Source: CAD feature listing. Evaluate the final solid. Frame: model axes, mm. A direction names the side the tool comes from. Give positions to 0.01 mm unless a question says otherwise; leave off trailing zeros. Write each loop counter-clockwise with the first axis right and the second up, starting at its lowest first coordinate (ties: lowest second). Pieces come first, ordered by that corner, then holes. Notation, with made-up numbers: (57, -23) -> (65, -23) arc R23 cw to (65, -14) -> close; hole circle Ø1 at (83.5, 21). An arc over 180 degrees is marked (long way). Answer as a JSON object with one key per item and string values. Group by question number.
Item 1: First-contact query: pin 1 Ø4 at (x, z) = (714, 304.5) entering from +Y; pin 2 Ø1.5 at (x, y) = (726, 437) entering from -Z; pin 3 Ø8 at (x, z) = (572, 173) entering from +Y. Flat tips, straight axial feed; report the tip coordinate or a pass-through.
Item 2: Access query for faces 1 (the face through (688.11, 629.81, -443.7)), 2 (the face through (687, 638, -900)). Directions: +Z, -Z, +X, -X, +Y, -Y. A direction counts if a zero-diameter tool reaches every point of the face in a straight line with its end or side. Return the directions, or none.
Item 3: Ray query, probe 1 along Z at (x, y) = (528, 589.5); probe 2 along Z at (x, y) = (235, 513.5); probe 3 along X at (y, z) = (640.5, -573.5). Return the intervals inside material, ascending. Write a range as from..to.
Item 4: Section query A-A on z = -118. Return the cut outline in (x, y), plus the area to 3 significant figures.
Autodesk Inventor part; units mm, degrees
ref_plane "end1" through (-1039.2305, 0, 0) normal (1, 0, 0) x (0, 1, 0)
ref_plane "end2" through (1039.2305, 0, 0) normal (1, 0, 0) x (0, 1, 0)
ref_plane "XZ Plane" through (0, 0, 0) normal (0, 1, 0) x (-1, 0, 0)
sketch "Sketch1" plane through (0, 0, 0) normal (0, 0, 1) x (1, 0, 0)
  arc A0 (0, 900) -> (-1039.2305, 0) centre (0, -150) ccw
  arc A1 (1039.2305, 0) -> (0, 900) centre (0, -150) ccw
  arc A2 (0, 890) -> (-1029.1258, 0) centre (0, -150) ccw
  arc A3 (1029.1258, 0) -> (0, 890) centre (0, -150) ccw
  line L0 (1029.1258, 0) -> (1039.2305, 0)
  line L1 (-1039.2305, 0) -> (-1029.1258, 0)
  point P0 (0, 0)
  dimension "d0" = 0
  dimension "d1" = 0
  dimension "d2" = 0
  dimension "d3" = 150
  dimension "d6" = 900
  dimension "d8" = 1039.2305
  dimension "d10" = 0
  dimension "d11" = 10
  dimension "d12" = 0
revolve "Revolution2" add sketch "Sketch1" angle 90 about axis through (1029.1258, 0, 0) along (1, 0, 0)
ref_plane "end1" through (-1039.2305, 0, 0) normal (1, 0, 0) x (0, 1, 0)
sketch "Sketch3" plane through (-1039.2305, 0, 0) normal (1, 0, 0) x (0, 1, 0)
  line L0 (900, 0) -> (0, 0)
  line L1 (0, 900) -> (0, 0)
  line L2 (900, 0) -> (0, 0)
  line L3 (0, 0) -> (0, 900)
  line L4 (0, 900) -> (900, 900)
  line L5 (900, 900) -> (900, 0)
extrude "Extrusion1" cut sketch "Sketch3" along normal blind 1039.2305
ref_plane "end2" through (1039.2305, 0, 0) normal (1, 0, 0) x (0, 1, 0)
sketch "Sketch4" plane through (0, -150, 0) normal (0, 0, -1) x (-0.7559289, 0.6546537, 0)
  arc A0 (687.3864, 793.7254) -> (-687.3864, 793.7254) centre (0, 0) ccw
  arc A1 (680.8398, 786.1661) -> (-679.748, 787.1104) centre (0, 0) ccw
  line L0 (680.8398, 786.1661) -> (687.3864, 793.7254)
  line L1 (-679.748, 787.1104) -> (-687.3864, 793.7254)
  point P0 (98.1981, 113.3893)
extrude "Extrusion2" add sketch "Sketch4" along normal blind 900
equation "\"d14\" = d8"
properties part number "cover2_sule_extended"
Worked answers:
{
 "1": {"pin 1": "y = 542.33", "pin 2": "z = 401.95", "pin 3": "y = 712.57"},
 "2": {"face 1": "-Z, -X, -Y", "face 2": "-Z, +X, -X, +Y, -Y"},
 "3": {"probe 1": "457.17..475.85", "probe 2": "693.73..706.46", "probe 3": "675.8..691.09"},
 "4": {"outline": "(0, 890) arc R1040 cw to (1029.13, 0) -> (1039.23, 0) arc R1050 ccw to (0, 900) -> close", "area": "14,900 mm^2"}
}
